```python
from build123d import *

# Parameters (mm, degrees)
F0_R     = 25.4
F0_R_2   = 6.35
F1_DEPTH = 6.35
F3_DEPTH = 6.351


with BuildPart() as f1:
    # F0 (on Front) → F1 (new body)
    with BuildSketch(Plane.XZ):
        Circle(F0_R)
        Circle(F0_R_2, mode=Mode.SUBTRACT)
    extrude(amount=F1_DEPTH)

    # F2 (on face) → F3 (cut, through all)
    with BuildSketch(Plane.XZ.offset(6.35)):
        with BuildLine():
            ThreePointArc((-5.6520317225, 24.7631689694), (-2.8552519313, 22.7872201957), (-0.6324557251, 25.3921247586))
            ThreePointArc((-0.6324557251, 25.3921247586), (-3.157941096, 25.2029245929), (-5.6520317225, 24.7631689694))
        make_face()
        with BuildLine():
            ThreePointArc((5.0336805768, 24.8962258154), (2.5294133993, 25.2737426563), (0, 25.4))
            ThreePointArc((0, 25.4), (2.286968716, 22.8512503362), (5.0336805768, 24.8962258154))
        make_face()
        with BuildLine():
            ThreePointArc((24.8962258154, -5.0336805768), (25.2737426563, -2.5294133993), (25.4, 0))
            ThreePointArc((25.4, 0), (22.8512503362, -2.286968716), (24.8962258154, -5.0336805768))
        make_face()
        with BuildLine():
            ThreePointArc((23.1519261522, -10.4474071158), (24.0772297289, -8.0899325449), (24.7631689694, -5.6520317225))
            ThreePointArc((24.7631689694, -5.6520317225), (21.7694233664, -7.3145112024), (23.1519261522, -10.4474071158))
        make_face()
        with BuildLine():
            ThreePointArc((20.2466922377, -15.3372570374), (21.6733839652, -13.244788692), (22.8846092447, -11.0206469736))
            ThreePointArc((22.8846092447, -11.0206469736), (19.5959866078, -11.9752735544), (20.2466922377, -15.3372570374))
        make_face()
        with BuildLine():
            ThreePointArc((16.3262046316, -19.4580328483), (18.1827442293, -17.7354958288), (19.8585196547, -15.8366409672))
            ThreePointArc((19.8585196547, -15.8366409672), (16.439925255, -16.035545686), (16.3262046316, -19.4580328483))
        make_face()
        with BuildLine():
            ThreePointArc((11.587052953, -22.6031016426), (13.7803457732, -21.3368711476), (15.8366409672, -19.8585196547))
            ThreePointArc((15.8366409672, -19.8585196547), (12.4594974028, -19.2917285982), (11.587052953, -22.6031016426))
        make_face()
        with BuildLine():
            ThreePointArc((6.266878056, -24.6147565381), (8.6869432384, -23.8683266521), (11.0206469736, -22.8846092447))
            ThreePointArc((11.0206469736, -22.8846092447), (7.8542983244, -21.5805436833), (6.266878056, -24.6147565381))
        make_face()
        with BuildLine():
            ThreePointArc((0.6324557251, -25.3921247586), (3.157941096, -25.2029245929), (5.6520317225, -24.7631689694))
            ThreePointArc((5.6520317225, -24.7631689694), (2.8552519313, -22.7872201957), (0.6324557251, -25.3921247586))
        make_face()
        with BuildLine():
            ThreePointArc((0, -25.4), (-2.286968716, -22.8512503362), (-5.0336805768, -24.8962258154))
            ThreePointArc((-5.0336805768, -24.8962258154), (-2.5294133993, -25.2737426563), (0, -25.4))
        make_face()
        with BuildLine():
            ThreePointArc((-5.6520317225, -24.7631689694), (-7.3145112024, -21.7694233664), (-10.4474071158, -23.1519261522))
            ThreePointArc((-10.4474071158, -23.1519261522), (-8.0899325449, -24.0772297289), (-5.6520317225, -24.7631689694))
        make_face()
        with BuildLine():
            ThreePointArc((-11.0206469736, -22.8846092447), (-11.9752735544, -19.5959866078), (-15.3372570374, -20.2466922377))
            ThreePointArc((-15.3372570374, -20.2466922377), (-13.244788692, -21.6733839652), (-11.0206469736, -22.8846092447))
        make_face()
        with BuildLine():
            ThreePointArc((-15.8366409672, -19.8585196547), (-16.035545686, -16.439925255), (-19.4580328483, -16.3262046316))
            ThreePointArc((-19.4580328483, -16.3262046316), (-17.7354958288, -18.1827442293), (-15.8366409672, -19.8585196547))
        make_face()
        with BuildLine():
            ThreePointArc((-19.8585196547, -15.8366409672), (-19.2917285982, -12.4594974028), (-22.6031016426, -11.587052953))
            ThreePointArc((-22.6031016426, -11.587052953), (-21.3368711476, -13.7803457732), (-19.8585196547, -15.8366409672))
        make_face()
        with BuildLine():
            ThreePointArc((-22.8846092447, -11.0206469736), (-21.5805436833, -7.8542983244), (-24.6147565381, -6.266878056))
            ThreePointArc((-24.6147565381, -6.266878056), (-23.8683266521, -8.6869432384), (-22.8846092447, -11.0206469736))
        make_face()
        with BuildLine():
            ThreePointArc((-24.7631689694, -5.6520317225), (-22.7872201957, -2.8552519313), (-25.3921247586, -0.6324557251))
            ThreePointArc((-25.3921247586, -0.6324557251), (-25.2029245929, -3.157941096), (-24.7631689694, -5.6520317225))
        make_face()
        with BuildLine():
            ThreePointArc((-25.4, 0), (-22.8512503362, 2.286968716), (-24.8962258154, 5.0336805768))
            ThreePointArc((-24.8962258154, 5.0336805768), (-25.2737426563, 2.5294133993), (-25.4, 0))
        make_face()
        with BuildLine():
            ThreePointArc((-24.7631689694, 5.6520317225), (-21.7694233664, 7.3145112024), (-23.1519261522, 10.4474071158))
            ThreePointArc((-23.1519261522, 10.4474071158), (-24.0772297289, 8.0899325449), (-24.7631689694, 5.6520317225))
        make_face()
        with BuildLine():
            ThreePointArc((-22.8846092447, 11.0206469736), (-19.5959866078, 11.9752735544), (-20.2466922377, 15.3372570374))
            ThreePointArc((-20.2466922377, 15.3372570374), (-21.6733839652, 13.244788692), (-22.8846092447, 11.0206469736))
        make_face()
        with BuildLine():
            ThreePointArc((-19.8585196547, 15.8366409672), (-16.439925255, 16.035545686), (-16.3262046316, 19.4580328483))
            ThreePointArc((-16.3262046316, 19.4580328483), (-18.1827442293, 17.7354958288), (-19.8585196547, 15.8366409672))
        make_face()
        with BuildLine():
            ThreePointArc((-15.8366409672, 19.8585196547), (-12.4594974028, 19.2917285982), (-11.587052953, 22.6031016426))
            ThreePointArc((-11.587052953, 22.6031016426), (-13.7803457732, 21.3368711476), (-15.8366409672, 19.8585196547))
        make_face()
        with BuildLine():
            ThreePointArc((-11.0206469736, 22.8846092447), (-7.8542983244, 21.5805436833), (-6.266878056, 24.6147565381))
            ThreePointArc((-6.266878056, 24.6147565381), (-8.6869432384, 23.8683266521), (-11.0206469736, 22.8846092447))
        make_face()
        with BuildLine():
            ThreePointArc((10.4474071158, 23.1519261522), (8.0899325449, 24.0772297289), (5.6520317225, 24.7631689694))
            ThreePointArc((5.6520317225, 24.7631689694), (7.3145112024, 21.7694233664), (10.4474071158, 23.1519261522))
        make_face()
        with BuildLine():
            ThreePointArc((15.3372570374, 20.2466922377), (13.244788692, 21.6733839652), (11.0206469736, 22.8846092447))
            ThreePointArc((11.0206469736, 22.8846092447), (11.9752735544, 19.5959866078), (15.3372570374, 20.2466922377))
        make_face()
        with BuildLine():
            ThreePointArc((19.4580328483, 16.3262046316), (17.7354958288, 18.1827442293), (15.8366409672, 19.8585196547))
            ThreePointArc((15.8366409672, 19.8585196547), (16.035545686, 16.439925255), (19.4580328483, 16.3262046316))
        make_face()
        with BuildLine():
            ThreePointArc((22.6031016426, 11.587052953), (21.3368711476, 13.7803457732), (19.8585196547, 15.8366409672))
            ThreePointArc((19.8585196547, 15.8366409672), (19.2917285982, 12.4594974028), (22.6031016426, 11.587052953))
        make_face()
        with BuildLine():
            ThreePointArc((24.6147565381, 6.266878056), (23.8683266521, 8.6869432384), (22.8846092447, 11.0206469736))
            ThreePointArc((22.8846092447, 11.0206469736), (21.5805436833, 7.8542983244), (24.6147565381, 6.266878056))
        make_face()
        with BuildLine():
            ThreePointArc((25.3921247586, 0.6324557251), (25.2029245929, 3.157941096), (24.7631689694, 5.6520317225))
            ThreePointArc((24.7631689694, 5.6520317225), (22.7872201957, 2.8552519313), (25.3921247586, 0.6324557251))
        make_face()
    extrude(amount=-F3_DEPTH, mode=Mode.SUBTRACT)


solid = f1.part
```
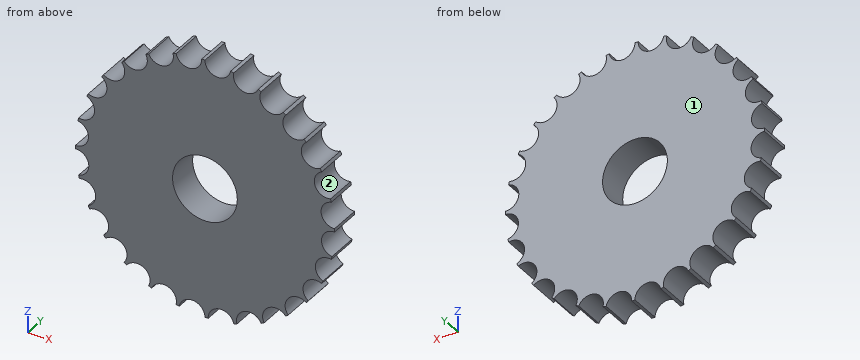
Work out the finished part from the listing and answer in its coordinate system (mm). Face numbers are marked on the shaded views. Round coordinates to 2 decimals unless told otherwise and drop trailing zeros. Write each loop counter-clockwise with the first axis right and the second up, starting at its lowest first coordinate (ties: lowest second). Pieces come first, ordered by that corner, then holes.
1) A cutting plane is placed at B-B on x = -7.5. Determine the outline of the cut face in (y, z), and give its area (3 significant figures).
2) Flat-ended cylindrical pins translate along their axes: P1, Ø1.5, axis at y = -0.5, z = 17, coming from the +X side; P2, Ø7.5, axis at x = 0, z = 0, coming from the -Y side; P3, Ø1, axis at x = 18, y = -4.5, coming from the -Z side; P4, Ø1.5, axis at x = -2, y = -2, coming from the +Z side. Find the tip coordinate at first contact, or state that the pin passes through.
3) Consider probe 1 along Z at (x, y) = (-3.5, -5.75); probe 2 along Z at (x, y) = (-0.5, -3); probe 3 along Z at (x, y) = (-18, -4.5). Determine where each line is inside the solid, lowest interval first.
4) Determine the mould class of the marked faces 1 and 2 for opening direction Z: pulls with the +Z half, pulls with the -Z half, needs draft (parallel to the pull), parting line crosses it, or undercut.
5) A cutting plane is placed at A-A on z = -3. Determine the outline of the cut face in (x, y), and give its area (3 significant figures).
Entries:
1. outline: (-6.35, -21.71) - (0, -21.71) - (0, 21.74) - (-6.35, 21.74) - close
1. area: 276 mm2
2. P1: stops at x = 19.52
2. P2: passes through
2. P3: stops at z = -15.38
2. P4: stops at z = 23.65
3. probe 1: z = -23.03 to -5.3, 5.3 to 22.79
3. probe 2: z = -23.87 to -6.33, 6.33 to 25.4
3. probe 3: z = -15.73 to 15.28
4. face 1: needs draft
4. face 2: undercut
5. outline: (-22.77, -6.35) - (-5.6, -6.35) - (-5.6, 0) - (-22.77, 0) - close; (5.6, -6.35) - (22.88, -6.35) - (22.88, 0) - (5.6, 0) - close
5. area: 219 mm2
